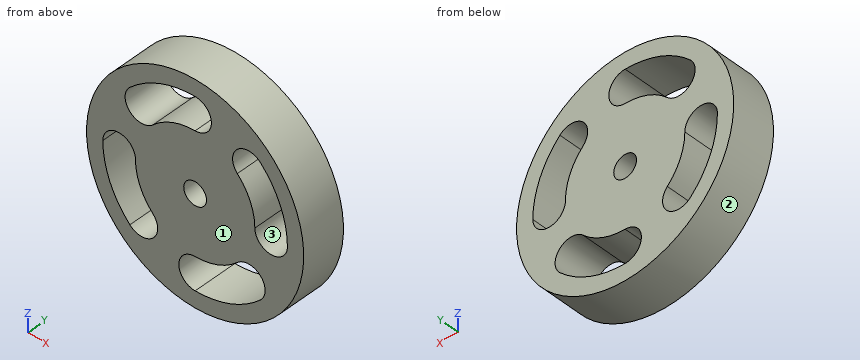
from build123d import *

# Parameters (mm, degrees)
SKETCH_1_R          = 50
EXTRUDE_1_DEPTH     = 20
SKETCH_2_R          = 5.25
CUT_EXTRUDE_1_DEPTH = 20
CUT_EXTRUDE_2_DEPTH = 20


with BuildPart() as part:
    # 草图1 → 凸台-拉伸1 (new body)
    with BuildSketch(Plane(origin=(0, 0, 0), x_dir=(1, 0, 0), z_dir=(0, 1, 0))):
        with Locations(Location((0, 0, 0), (0, 0, 270))):
            Circle(SKETCH_1_R)
    extrude(amount=EXTRUDE_1_DEPTH)

    # 草图2 → 切除-拉伸1 (cut)
    with BuildSketch(Plane(origin=(0, 20, 0), x_dir=(1, 0, 0), z_dir=(0, 1, 0))):
        with Locations(Location((0, 0, 0), (0, 0, 270))):
            Circle(SKETCH_2_R)
    extrude(amount=-CUT_EXTRUDE_1_DEPTH, mode=Mode.SUBTRACT)

    # 草图3 → 切除-拉伸2 (cut)
    with BuildSketch(Plane(origin=(0, 20, 0), x_dir=(1, 0, 0), z_dir=(0, 1, 0))):
        with BuildLine():
            ThreePointArc((42.5, 0), (35, 7.5), (27.5, 0))
            ThreePointArc((27.5, 0), (25.406687144, -10.52379439), (19.445436483, -19.445436483))
            ThreePointArc((19.445436483, -19.445436483), (19.445436477, -30.052038195), (30.052038189, -30.052038212))
            ThreePointArc((30.052038189, -30.052038212), (39.264880129, -16.264045883), (42.5, 0))
        make_face()
        with BuildLine():
            ThreePointArc((2e-09, 27.5), (10.523794391, 25.406687144), (19.445436483, 19.445436483))
            ThreePointArc((19.445436483, 19.445436483), (30.0520382, 19.445436483), (30.0520382, 30.0520382))
            ThreePointArc((30.0520382, 30.0520382), (16.264045902, 39.264880121), (5.8e-08, 42.5))
            ThreePointArc((5.8e-08, 42.5), (-7.5, 35.000000028), (2e-09, 27.5))
        make_face()
        with BuildLine():
            ThreePointArc((-30.0520382, -30.0520382), (-16.264045799, -39.264880163), (1.65e-07, -42.5))
            ThreePointArc((1.65e-07, -42.5), (7.5, -34.999999948), (6.1e-08, -27.5))
            ThreePointArc((6.1e-08, -27.5), (-10.523794348, -25.406687162), (-19.44543646, -19.445436505))
            ThreePointArc((-19.44543646, -19.445436505), (-30.052038189, -19.445436472), (-30.0520382, -30.0520382))
        make_face()
        with BuildLine():
            ThreePointArc((-27.5, 0), (-25.406687154, 10.523794365), (-19.445436521, 19.445436445))
            ThreePointArc((-19.445436521, 19.445436445), (-19.445436492, 30.05203821), (-30.052038258, 30.052038143))
            ThreePointArc((-30.052038258, 30.052038143), (-39.264880164, 16.264045797), (-42.5, -8.9e-08))
            ThreePointArc((-42.5, -8.9e-08), (-34.999999956, -7.5), (-27.5, 0))
        make_face()
    extrude(amount=-CUT_EXTRUDE_2_DEPTH, mode=Mode.SUBTRACT)


solid = part.part
Check sheet for the modelled part. Datum: model origin and axes. Units: mm. Face numbers are marked on the shaded views. Coordinates: 2 decimals unless noted, no trailing zeros. Loops run counter-clockwise (first coordinate to the right, second up) from the corner with the lowest first, then second, coordinate; pieces in that order, holes last. Notation, with made-up numbers: (47.5, 58.25) -> (105.5, 58.25) arc R25 ccw to (105.5, 94.25) -> close; hole circle Ø7 at (62, 29). An arc over 180 degrees is marked (long way). Answer in a Markdown table with one row per item.
1. Release check for a two-part mould opening along X. For the marked faces 1, 2 and 3 record: released by +X, released by -X, zero draft, split by the parting line, or undercut.
Check values:
| item | result |
|---|---|
| face 1 | zero draft |
| face 2 | split by the parting line |
| face 3 | undercut |
2. Sectioned sample at B-B, the plane x = -37. Record the boundary of the cut face in (y, z).
Check values:
| item | result |
|---|---|
| outline | (0, -33.63) -> (20, -33.63) -> (20, -20.91) -> (0, -20.91) -> close; (0, 7.23) -> (20, 7.23) -> (20, 33.63) -> (0, 33.63) -> close |
3. Sectioned sample at C-C, the plane y = 6.25. Record the boundary of the cut face in (x, z).
Check values:
| item | result |
|---|---|
| outline | circle Ø100 at (0, 0); hole (-42.5, 0) arc R42.5 ccw to (-30.05, -30.05) arc R7.5 ccw to (-19.45, -19.45) arc R27.5 cw to (-27.5, 0) arc R7.5 ccw to start; hole (-30.05, 30.05) arc R7.5 ccw to (-19.45, 19.45) arc R27.5 cw to (0, 27.5) arc R7.5 ccw to (0, 42.5) arc R42.5 ccw to start; hole circle Ø10.5 at (0, 0); hole (0, -42.5) arc R42.5 ccw to (30.05, -30.05) arc R7.5 ccw to (19.45, -19.45) arc R27.5 cw to (0, -27.5) arc R7.5 ccw to start; hole (19.45, 19.45) arc R27.5 cw to (27.5, 0) arc R7.5 ccw to (42.5, 0) arc R42.5 ccw to (30.05, 30.05) arc R7.5 ccw to start |
4. Go/stop test with flat-tipped pins: pin 1 (1 mm diameter, centred on y = 5, z = -38, fed in from +X); pin 2 (4 mm diameter, centred on y = 12.5, z = -35.5, fed in from +X); pin 3 (1.5 mm diameter, centred on x = 10, y = 16, fed in from +Z). Record where each tip stops, or that it passes through.
Check values:
| item | result |
|---|---|
| pin 1 | stops at x = 33.07 |
| pin 2 | stops at x = 37.12 |
| pin 3 | stops at z = 49.14 |
5. Sectioned sample at D-D, the plane x = -1.5. Record the boundary of the cut face in (y, z).
Check values:
| item | result |
|---|---|
| outline | (0, -49.98) -> (20, -49.98) -> (20, -42.35) -> (0, -42.35) -> close; (0, -27.65) -> (20, -27.65) -> (20, -5.03) -> (0, -5.03) -> close; (0, 5.03) -> (20, 5.03) -> (20, 27.46) -> (0, 27.46) -> close; (0, 42.47) -> (20, 42.47) -> (20, 49.98) -> (0, 49.98) -> close |
6. Material ranges on line 1 along Z through (x, y) = (-4.5, 6.5); line 2 along X through (y, z) = (10.5, 31), recorded low to high. Write a range as [from, to].
Check values:
| item | result |
|---|---|
| line 1 | z = [-49.8, -41], [-29, -2.7], [2.7, 27.13], [42.26, 49.8] |
| line 2 | x = [-39.23, -29.07], [6.34, 20.6], [28.89, 39.23] |
7. Sectioned sample at A-A, the plane z = -35. Record the boundary of the cut face in (x, y).
Check values:
| item | result |
|---|---|
| outline | (-35.71, 0) -> (-7.5, 0) -> (-7.5, 20) -> (-35.71, 20) -> close; (24.11, 0) -> (35.71, 0) -> (35.71, 20) -> (24.11, 20) -> close |
